Could you check a few things on this model? Use its own coordinates, in mm. Coordinates: 2 decimals unless noted, no trailing zeros. Loops run counter-clockwise (first coordinate to the right, second up) from the corner with the lowest first, then second, coordinate; pieces in that order, holes last. Notation, with made-up numbers: (60.5, 61) - (103.5, 61) arc R13 cw to (103.5, 65) - close; hole circle Ø5 at (-37.75, -11). An arc over 180 degrees is marked (long way). Use CSV: the item, a comma, the result in double quotes.
from build123d import *

# Parameters (mm, degrees)
SKETCH1_R           = 79
SKETCH1_R_2         = 3
SKETCH1_R_3         = 5
BOSS_EXTRUDE1_DEPTH = 1.5875


with BuildPart() as part:
    # Sketch1 → Boss-Extrude1 (new body)
    with BuildSketch(Plane(origin=(0, 0, 0), x_dir=(1, 0, 0), z_dir=(0, 1, 0))):
        Circle(SKETCH1_R)
        with Locations((0, 66.2)):
            Circle(SKETCH1_R_2, mode=Mode.SUBTRACT)
        with Locations((66.2, 0)):
            Circle(SKETCH1_R_2, mode=Mode.SUBTRACT)
        with Locations((0, -66.2)):
            Circle(SKETCH1_R_2, mode=Mode.SUBTRACT)
        with Locations((-66.2, 0)):
            Circle(SKETCH1_R_2, mode=Mode.SUBTRACT)
        Circle(SKETCH1_R_3, mode=Mode.SUBTRACT)
    extrude(amount=BOSS_EXTRUDE1_DEPTH)


solid = part.part
(1) Please list where these lines run through material, in increasing order: line 1 (X direction, y = 0.95, z = 0); line 2 (X direction, y = 0.7, z = -66.2).
Computed:
line 1,"x = -79 to -69.2, -63.2 to -5, 5 to 63.2, 69.2 to 79"
line 2,"x = -43.11 to -3, 3 to 43.11"
(2) Thinking about a two-plate mould opening in Z: for faces 1 (the face through (-1, 1.588, 16)), 2 (the face through (63.2, 0.8, -0.1)), 3 (the face through (-58.23, 0.78, -53.39)), which applies, +Z half, -Z half, draft (parallel to the pull), parting line (faces both ways), or undercut?
Computed:
face 1,"draft"
face 2,"undercut"
face 3,"parting line"
(3) Suppose I cut it at D-D (y = 0.4). Write out the boundary of the cut face in (x, z).
Computed:
outline,"circle Ø158 at (0, 0); hole circle Ø6 at (-66.2, 0); hole circle Ø10 at (0, 0); hole circle Ø6 at (0, -66.2); hole circle Ø6 at (0, 66.2); hole circle Ø6 at (66.2, 0)"
(4) Suppose I cut it at C-C (z = 66.2). Write out the boundary of the cut face in (x, y), plus the area to 3 significant figures.
Computed:
outline,"(-43.11, 0) - (-3, 0) - (-3, 1.59) - (-43.11, 1.59) - close; (3, 0) - (43.11, 0) - (43.11, 1.59) - (3, 1.59) - close"
area,"127 mm²"
(5) Suppose I cut it at A-A (z = 0). Write out the boundary of the cut face in (x, y), plus the area to 3 significant figures.
Computed:
outline,"(-79, 0) - (-69.2, 0) - (-69.2, 1.59) - (-79, 1.59) - close; (-63.2, 0) - (-5, 0) - (-5, 1.59) - (-63.2, 1.59) - close; (5, 0) - (63.2, 0) - (63.2, 1.59) - (5, 1.59) - close; (69.2, 0) - (79, 0) - (79, 1.59) - (69.2, 1.59) - close"
area,"216 mm²"
(6) Suppose I cut it at B-B (x = 0). Write out the boundary of the cut face in (y, z).
Computed:
outline,"(0, -79) - (1.59, -79) - (1.59, -69.2) - (0, -69.2) - close; (0, -63.2) - (1.59, -63.2) - (1.59, -5) - (0, -5) - close; (0, 5) - (1.59, 5) - (1.59, 63.2) - (0, 63.2) - close; (0, 69.2) - (1.59, 69.2) - (1.59, 79) - (0, 79) - close"
